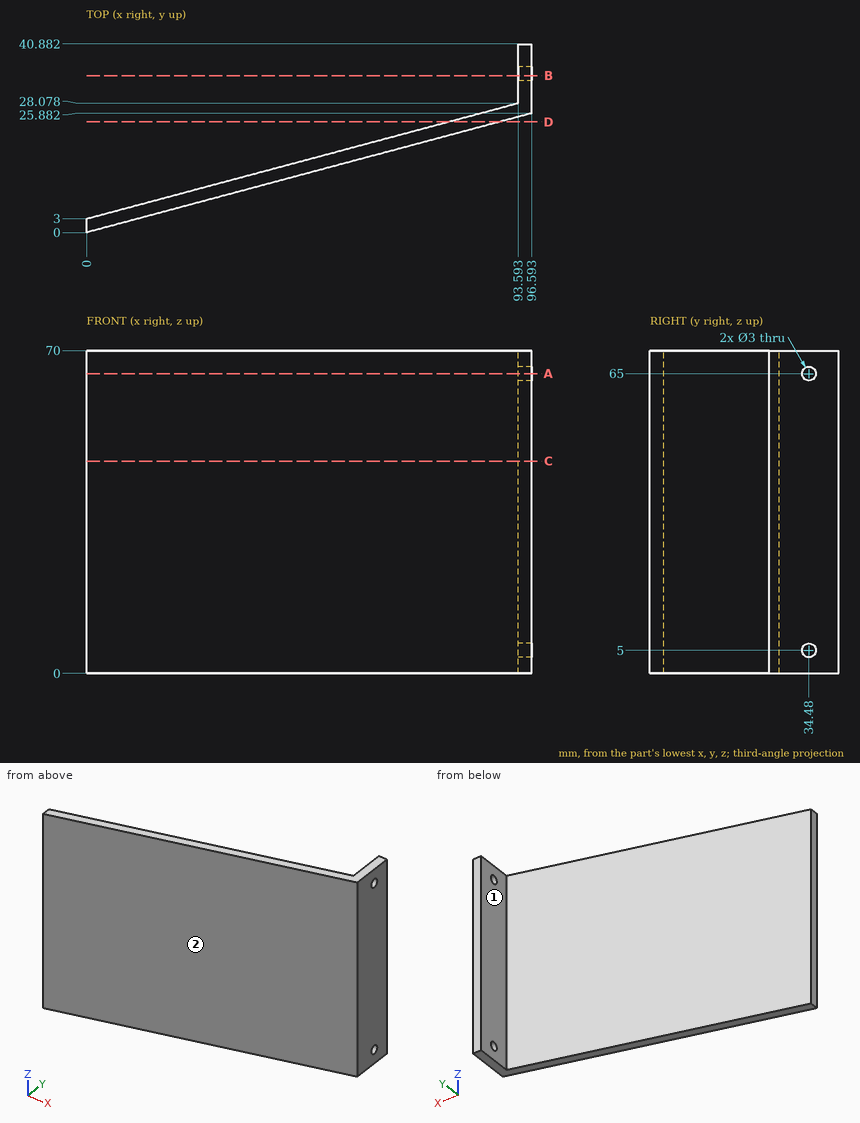
Answer from the drawing. Dimensions are ordinates in mm from the lowest x, y and z of the part. A direction names the side the tool comes from. Round coordinates to 2 decimals unless told otherwise and drop trailing zeros. Write each loop counter-clockwise with the first axis right and the second up, starting at its lowest first coordinate (ties: lowest second). Pieces come first, ordered by that corner, then holes. Notation, with made-up numbers: M 8.25,-37.75 L 37.25,-37.75 A35 ccw 37.25,1.25 Z; hole C -30,83.5 d8. An arc over 180 degrees is marked long. Write each question's results on one line, items separated by ' | '. Start each with the question number.
Item 1: A cutting plane is placed at D-D on y = 24. Write down the section's boundary in (x, z).
Item 2: A cutting plane is placed at A-A on z = 65. Write down the section's boundary in (x, y), and give its area (3 significant figures).
Item 3: A cutting plane is placed at B-B on y = 34. Write down the section's boundary in (x, z).
Item 4: Flat-ended cylindrical pins translate along their axes: pin 1 Ø6 at (x, z) = (15.5, 62.5) entering from +Y; pin 2 Ø4 at (y, z) = (37, 36) entering from -X; pin 3 Ø5 at (x, z) = (77.5, 24) entering from +Y. Find the tip coordinate at first contact, or state that the pin passes through.
Item 5: A cutting plane is placed at C-C on z = 46. Write down the section's boundary in (x, y), and give its area (3 significant figures).
Item 6: For the marked faces 1 and 2, determine the directions among +Z, -Z, +X, -X, +Y, -Y from which every point of the face is accessible in a straight line to the end or side of a thin tool.
Item 7: Straight lines are drawn through the part: L1, parallel to X at y = 37.5, z = 51.5; L2, parallel to Y at x = 94, z = 65; L3, parallel to Y at x = 95.05, z = 65. For each, find the intervals that lie inside material, in ascending order. Write a range as [from, to].
Check sheet entries:
1) outline: M 78.37,0 L 89.57,0 L 89.57,70 L 78.37,70 Z
2) outline: M 0,0 L 96.59,25.88 L 96.59,32.98 L 93.59,32.98 L 93.59,28.08 L 0,3 Z; M 93.59,35.98 L 96.59,35.98 L 96.59,40.88 L 93.59,40.88 Z | area: 318 mm²
3) outline: M 93.59,0 L 96.59,0 L 96.59,3.58 L 93.59,3.58 Z; M 93.59,6.42 L 96.59,6.42 L 96.59,63.58 L 93.59,63.58 Z; M 93.59,66.42 L 96.59,66.42 L 96.59,70 L 93.59,70 Z
4) pin 1: y = 7.96 | pin 2: x = 93.59 | pin 3: y = 24.44
5) outline: M 0,0 L 96.59,25.88 L 96.59,40.88 L 93.59,40.88 L 93.59,28.08 L 0,3 Z | area: 327 mm²
6) face 1: +Z, -Z, -X, +Y | face 2: +Z, -Z, +X, -Y
7) L1: [93.59, 96.59] | L2: [25.19, 32.98], [35.98, 40.88] | L3: [25.47, 32.98], [35.98, 40.88]
